Geometry: final body of the model. Coordinates: model frame, mm. A direction names the side the tool comes from. Give positions to 0.01 mm unless a question says otherwise; leave off trailing zeros. Loops run counter-clockwise (first coordinate to the right, second up) from the corner with the lowest first, then second, coordinate; pieces in that order, holes last. Notation, with made-up numbers: M 30.25,36 L 63.25,36 A32 ccw 63.25,73 Z; hole C 15,44.5 d6. An arc over 180 degrees is marked long. One line per question, with ' | ' between items. Start each with the question number.
from build123d import *

# Parameters (mm, degrees)
F0_R     = 37.5
F0_R_2   = 25
F1_DEPTH = 25
F2_W     = 5
F2_H     = 20
F3_DEPTH = 50
F2_W_2   = 75
F2_H_2   = 10
F4_DEPTH = 10
F5_DEPTH = 10
F2_R     = 5
F6_DEPTH = 37.501


with BuildPart() as f1:
    # F0 (on Front) → F1 (new body, symmetric)
    with BuildSketch(Plane.XZ):
        Circle(F0_R)
        Circle(F0_R_2, mode=Mode.SUBTRACT)
    extrude(amount=F1_DEPTH, both=True)

    # F2 (on Top) → F3 (cut, symmetric)
    with BuildSketch(Plane.XY):
        with Locations((-35, 0)):
            Rectangle(F2_W, F2_H)
        with Locations((35, 0)):
            Rectangle(F2_W, F2_H)
    extrude(amount=F3_DEPTH, both=True, mode=Mode.SUBTRACT)

    # F2 (on Top) → F4 (cut, symmetric)
    with BuildSketch(Plane.XY):
        with Locations((0, -20)):
            Rectangle(F2_W_2, F2_H_2)
    extrude(amount=F4_DEPTH, both=True, mode=Mode.SUBTRACT)

    # F2 (on Top) → F5 (cut, symmetric)
    with BuildSketch(Plane.XY):
        with Locations((0, -20)):
            Rectangle(F2_W_2, F2_H_2)
    extrude(amount=F5_DEPTH, both=True, mode=Mode.SUBTRACT)

    # F2 (on Top) → F6 (cut, through all)
    with BuildSketch(Plane.XY):
        Circle(F2_R)
    extrude(amount=F6_DEPTH, mode=Mode.SUBTRACT)


solid = f1.part
Q1. Material intervals for L1, parallel to Z at x = 0, y = 10; L2, parallel to Y at x = 34.5, z = -4.5; L3, parallel to X at y = -12.5, z = -8.5, sorted ascending.
Q2. Section A-A, the plane x = 0. Output: boundary loops of the cut face in (y, z).
Q3. Section C-C, the plane y = -20.5. Output: boundary loops of the cut face in (x, z), plus the area to 4 significant figures.
Q4. Draft query along Z for faces 1 (the flat face through (24, 25, -8)), 2 (the flat face through (30, -15, 0)), 3 (the cylindrical face through (-8.13, -0.35, -36.61)). Return one class per face: released by +Z, released by -Z, zero draft, split by the parting line, or undercut.
Q5. Contact query for flat-ended pins moving along their axis: pin 1 (4 mm diameter, centred on x = -35.5, z = 0, fed in from -Y); pin 2 (8 mm diameter, centred on x = 0, y = 0, fed in from -Z); pin 3 (10 mm diameter, centred on y = 7, z = -27, fed in from +X). Output: stop coordinate, or through.
Q6. Set-up query: faces 4 (the flat face through (-30, -15, 0)), 5 (the flat face through (-34, 10, 0)), 6 (the flat face through (34, -10, 0)). Return all of +Z, -Z, +X, -X, +Y, -Y with unobstructed straight access to the full face (end or side cutting, diameter ignored); none if empty.
Q7. Section D-D, the plane x = -17. Output: boundary loops of the cut face in (y, z).
Q8. Section B-B, the plane z = 0. Output: boundary loops of the cut face in (x, y), plus the area to 3 significant figures.
Model answer:
1) L1: z = -37.5 to -25, 25 to 37.5 | L2: y = -15 to -10, 10 to 25 | L3: x = -36.52 to -23.51, 23.51 to 36.52
2) outline: M -25,-37.5 L 25,-37.5 L 25,-25 L -25,-25 Z; M -25,25 L -5,25 L -5,37.5 L -25,37.5 Z; M 5,25 L 25,25 L 25,37.5 L 5,37.5 Z
3) outline: M -36.14,-10 A37.5 ccw 36.14,-10 L 22.91,-10 A25 cw -22.91,-10 Z; M -36.14,10 L -22.91,10 A25 cw 22.91,10 L 36.14,10 A37.5 ccw Z | area: 1,945 mm^2
4) face 1: zero draft | face 2: undercut | face 3: split by the parting line
5) pin 1: stops at y = -15 | pin 2: stops at z = -37.5 | pin 3: stops at x = 30.37
6) face 4: +X, -X, -Y | face 5: +Z, -Z, -X | face 6: +Z, -Z, +X
7) outline: M -25,-33.43 L 25,-33.43 L 25,-18.33 L -25,-18.33 Z; M -25,18.33 L 25,18.33 L 25,33.43 L -25,33.43 Z
8) outline: M -37.5,-15 L -25,-15 L -25,25 L -37.5,25 L -37.5,10 L -32.5,10 L -32.5,-10 L -37.5,-10 Z; M 25,-15 L 37.5,-15 L 37.5,-10 L 32.5,-10 L 32.5,10 L 37.5,10 L 37.5,25 L 25,25 Z | area: 800 mm^2
